```python
from build123d import *

# Parameters (mm, degrees)
PAD003_DEPTH    = 2
SKETCH003_R     = 3
SKETCH004_R     = 1.5
SKETCH005_R     = 3
SKETCH006_R     = 1.5
SKETCH007_R     = 3
SKETCH008_R     = 1.5
SKETCH001_R     = 3
SKETCH002_R     = 1.5
PAD_DEPTH       = 2
CHAMFER_SIZE    = 2
PAD004_DEPTH    = 2
PAD001_DEPTH    = 2
PAD002_DEPTH    = 2
SKETCH013_R     = 1.25
POCKET_DEPTH    = 83.001
SKETCH014_R     = 1.25
POCKET001_DEPTH = 83.001002


with BuildPart() as pad003:
    # Sketch011 → Pad003 (new body)
    with BuildSketch(Plane.YZ.offset(39.5)):
        Polygon((-21.5, 0), (21.5, 0), (21.5, 4), (10, 9), (-10, 9), (-21.5, 4), align=None)
    extrude(amount=PAD003_DEPTH)


with BuildPart() as loft001:
    # Sketch003 → Loft001 section 0
    with BuildSketch(Plane.XY):
        with Locations((35, -35)):
            Circle(SKETCH003_R)
    # Sketch004 → Loft001 section 1
    with BuildSketch(Plane.XY.offset(2)):
        with Locations((35, -35)):
            Circle(SKETCH004_R)
    loft(ruled=True)


with BuildPart() as loft002:
    # Sketch005 → Loft002 section 0
    with BuildSketch(Plane.XY):
        with Locations((-35, 35)):
            Circle(SKETCH005_R)
    # Sketch006 → Loft002 section 1
    with BuildSketch(Plane.XY.offset(2)):
        with Locations((-35, 35)):
            Circle(SKETCH006_R)
    loft(ruled=True)


with BuildPart() as loft003:
    # Sketch007 → Loft003 section 0
    with BuildSketch(Plane.XY):
        with Locations((35, 35)):
            Circle(SKETCH007_R)
    # Sketch008 → Loft003 section 1
    with BuildSketch(Plane.XY.offset(2)):
        with Locations((35, 35)):
            Circle(SKETCH008_R)
    loft(ruled=True)


with BuildPart() as loft_body:
    # Sketch001 → Loft section 0
    with BuildSketch(Plane.XY):
        with Locations((-35, -35)):
            Circle(SKETCH001_R)
    # Sketch002 → Loft section 1
    with BuildSketch(Plane.XY.offset(2)):
        with Locations((-35, -35)):
            Circle(SKETCH002_R)
    loft(ruled=True)


with BuildPart() as cut003:
    # Sketch → Pad (new body)
    with BuildSketch(Plane.XY):
        with BuildLine():
            Line((21.499998, -41.5), (-21.500002, -41.5))
            Line((-21.500002, -39), (-21.500002, -41.5))
            ThreePointArc((-21.500002, -39), (-22.000002, -38.5), (-22.500002, -39))
            Line((-22.500002, -41.5), (-22.500002, -39))
            Line((-22.500002, -41.5), (-41.500002, -41.5))
            Line((-41.500002, -41.5), (-41.500002, -22.5))
            Line((-39.000002, -22.5), (-41.500002, -22.5))
            ThreePointArc((-39.000002, -22.5), (-38.500001, -22.000001), (-39, -21.5))
            Line((-41.5, -21.5), (-39, -21.5))
            Line((-41.5, -21.5), (-41.5, 21.5))
            Line((-41.5, 21.5), (-39, 21.5))
            ThreePointArc((-39, 21.5), (-38.5, 22.000001), (-39.000002, 22.5))
            Line((-39.000002, 22.5), (-41.500002, 22.5))
            Line((-41.500002, 41.5), (-41.500002, 22.5))
            Line((-22.500002, 41.5), (-41.500002, 41.5))
            Line((-22.500002, 41.5), (-22.500002, 39))
            ThreePointArc((-22.500002, 39), (-22.000002, 38.5), (-21.500002, 39))
            Line((-21.500002, 39), (-21.500002, 41.5))
            Line((21.499998, 41.5), (-21.500002, 41.5))
            Line((21.499998, 39), (21.499998, 41.5))
            ThreePointArc((21.499998, 39), (21.999998, 38.5), (22.499998, 39))
            Line((22.499998, 41.5), (22.499998, 39))
            Line((22.499998, 41.5), (41.499998, 41.5))
            Line((41.499998, 41.5), (41.499998, 22.5))
            Line((38.999998, 22.5), (41.499998, 22.5))
            ThreePointArc((38.999998, 22.5), (38.499996, 21.999999), (39, 21.5))
            Line((41.5, 21.5), (39, 21.5))
            Line((41.5, -21.5), (41.5, 21.5))
            Line((41.5, -21.5), (39, -21.5))
            ThreePointArc((39, -21.5), (38.500002, -21.999999), (38.999998, -22.5))
            Line((38.999998, -22.5), (41.499998, -22.5))
            Line((41.499998, -41.5), (41.499998, -22.5))
            Line((22.499998, -41.5), (41.499998, -41.5))
            Line((22.499998, -41.5), (22.499998, -39))
            ThreePointArc((22.499998, -39), (21.999998, -38.5), (21.499998, -39))
            Line((21.499998, -39), (21.499998, -41.5))
        make_face()
    extrude(amount=PAD_DEPTH)

    # Chamfer
    chamfer_edges = [cut003.edges().sort_by_distance(p)[0] for p in [
        (-41.500002, -41.5, 1),
        (-41.500002, 41.5, 1),
        (41.499998, -41.5, 1),
        (41.499998, 41.5, 1),
    ]]
    chamfer(chamfer_edges, length=CHAMFER_SIZE)

    # Cut: cut Loft body
    add(loft_body.part, mode=Mode.SUBTRACT)

    # Cut001: cut Loft003
    add(loft003.part, mode=Mode.SUBTRACT)

    # Cut002: cut Loft002
    add(loft002.part, mode=Mode.SUBTRACT)

    # Cut003: cut Loft001
    add(loft001.part, mode=Mode.SUBTRACT)


with BuildPart() as fusion:
    # Sketch012 → Pad004 (new body)
    with BuildSketch(Plane.YZ.offset(-41.5)):
        Polygon((-21.5, 0), (21.5, 0), (21.5, 4), (10, 9), (-10, 9), (-21.5, 4), align=None)
    extrude(amount=PAD004_DEPTH)

    # Fusion: union Cut003
    add(cut003.part)


with BuildPart() as pad001:
    # Sketch009 → Pad001 (new body)
    with BuildSketch(Plane.XZ.offset(39.5)):
        Polygon((-21.5, 0), (21.5, 0), (21.5, 4), (10, 9), (-10, 9), (-21.5, 4), align=None)
    extrude(amount=PAD001_DEPTH)


with BuildPart() as pocket001:
    # Sketch010 → Pad002 (new body)
    with BuildSketch(Plane.XZ.offset(-41.5)):
        Polygon((-21.5, 0), (21.5, 0), (21.5, 4), (10, 9), (-10, 9), (-21.5, 4), align=None)
    extrude(amount=PAD002_DEPTH)

    # Fusion001: union Pad003, Fusion, Pad001
    add(pad003.part)
    add(fusion.part)
    add(pad001.part)

    # Sketch013 → Pocket (cut, through all)
    with BuildSketch(Plane.XZ.offset(41.5)):
        with Locations((0, 4.5)):
            Circle(SKETCH013_R)
    extrude(amount=-POCKET_DEPTH, mode=Mode.SUBTRACT)

    # Sketch014 → Pocket001 (cut, through all)
    with BuildSketch(Plane.YZ.offset(41.5)):
        with Locations((0, 4.5)):
            Circle(SKETCH014_R)
    extrude(amount=-POCKET001_DEPTH, mode=Mode.SUBTRACT)


solid = pocket001.part
```
Check sheet for the modelled part. Datum: model origin and axes. Units: mm. A direction names the side the tool comes from. Give positions to 0.01 mm unless a question says otherwise; leave off trailing zeros. Write each loop counter-clockwise with the first axis right and the second up, starting at its lowest first coordinate (ties: lowest second). Pieces come first, ordered by that corner, then holes. Notation, with made-up numbers: (27, -24) -> (73, -24) arc R20 cw to (73, -19) -> close; hole circle Ø2 at (0.25, 44.5). An arc over 180 degrees is marked (long way). Use CSV: the item, a comma, the result in double quotes. Start each with the question number.
Q1. Depth check by flat-ended pin: P1, Ø0.6, axis at x = -40, z = 1, coming from the -Y side; P2, Ø0.6, axis at x = -40.5, z = 1, coming from the +Y side; P3, Ø4, axis at y = -20, z = 7, coming from the +X side; P4, Ø1, axis at y = 40.5, z = 1.5, coming from the +X side. Enter the tip coordinate at first touch or a pass-through.
Q2. Cross-section at C-C on z = 7.25. Enter the section's corners in (x, y) (3 decimals), and give its area (3 significant figures).
Q3. Tool access check on faces 4 (the flat face through (-21.5, -40, 1)), 5 (the flat face through (40, 21.5, 2)), 6 (the flat face through (22.5, 40, 1)). Record the directions out of +Z, -Z, +X, -X, +Y, -Y that give a thin tool (end or side, any length) a straight path to the whole face; none if there is none.
Q4. Cross-section at D-D on y = -35. Count the separate pieces of the cut face and the enclosed holes in it, and give its area (3 significant figures).
Q5. Release check for a two-part mould opening along X. For faces 1 (the flat face through (15.83, -40.486, 6.465)), 2 (the flat face through (0, -39.5, 7)), 3 (the cylindrical face through (-0.27, -40.51, 3.28)) record: +X half, -X half, draft (parallel to the pull), parting line (faces both ways), or undercut.
Q6. Scan lines: line 1 along X through (y, z) = (-16.5, 5); line 2 along Z through (x, y) = (-40.6, 0). Record each from-to range of solid material in increasing order.
Q7. Cross-section at A-A on x = 3. Enter the section's corners in (y, z), and give its area (3 significant figures).
Working result:
1,P1,"stops at y = -41.3"
1,P2,"stops at y = 40.8"
1,P3,"passes through"
1,P4,"stops at x = 41"
2,outline,"(-41.5, -14.025) -> (-39.5, -14.025) -> (-39.5, 14.025) -> (-41.5, 14.025) -> close; (-14.025, -41.5) -> (14.025, -41.5) -> (14.025, -39.5) -> (-14.025, -39.5) -> close; (-14.025, 39.5) -> (14.025, 39.5) -> (14.025, 41.5) -> (-14.025, 41.5) -> close; (39.5, -14.025) -> (41.5, -14.025) -> (41.5, 14.025) -> (39.5, 14.025) -> close"
2,area,"224 mm^2"
3,face 4,"+Z, -Z, -Y"
3,face 5,"+Z, -Z, +X"
3,face 6,"+Z, -Z, +Y"
4,separate pieces,"3"
4,enclosed holes,"0"
4,area,"148 mm^2"
5,face 1,"+X half"
5,face 2,"draft"
5,face 3,"undercut"
6,line 1,"x = -41.5 to -39.5, 39.5 to 41.5"
6,line 2,"z = 0 to 3.25, 5.75 to 9"
7,outline,"(-41.5, 0) -> (41.5, 0) -> (41.5, 9) -> (39.5, 9) -> (39.5, 2) -> (-39.5, 2) -> (-39.5, 9) -> (-41.5, 9) -> close"
7,area,"194 mm^2"
